The listing builds one solid part. Answer for the finished solid, in the listing's coordinates (mm). A direction names the side the tool comes from. Coordinates: 2 decimals unless noted, no trailing zeros. Order: outer loops, then holes, each group sorted by start corner. A loop starts at its lowest first (then second) coordinate and runs counter-clockwise, first axis right, second up. Notation, with made-up numbers: (24, -6) -> (34, -6) arc R10 ccw to (34, 10) -> close; hole circle Ø1 at (54.5, 16). An arc over 180 degrees is marked (long way). Write each question's results on one line, items separated by ' | '. Start each with the question number.
(1) Determine the mould class of faces 5 (the face through (10.75, -1.97, -25.84)), 6 (the face through (-10, 45, -205)), 7 (the face through (-5, -2, -169)), 8 (the face through (-33, -1, -126)) for opening direction X: +X half, -X half, draft (parallel to the pull), parting line (faces both ways), or undercut.
(2) A tool of negligible diameter and unlimited length cuts with its end or side. For faces 1 (the face through (-10, -2, -205)), 2 (the face through (3, 4, -207)), 3 (the face through (-5, -2, -13)), 4 (the face through (10.75, -1.97, -181.84)), from which of +Z, -Z, +X, -X, +Y, -Y can it reach the whole face along a straight path? Write none if from no direction.
(3) The part is cut by section D-D, the plane x = -17. Give the vertices of the cut face in (y, z).
(4) Given pin 1 (1.5 mm diameter, centred on x = -5.5, y = 38.5, fed in from +Z); pin 2 (6 mm diameter, centred on x = -15, z = -99, fed in from +Y), each flat-ended and moving along its own axis, determine where each tip first touches the part or whether it passes through.
(5) The part is cut by section C-C, the plane z = -66. Give the vertices of the cut face in (x, y).
(6) Straight lines are drawn through the part: L1, parallel to Y at x = 0, z = -200; L2, parallel to X at y = -3, z = 0; L3, parallel to Z at x = -6.5, y = 14. For each, find the intervals that lie inside material, in ascending order.
(7) The part is cut by section B-B, the plane y = 14. Give the vertices of the cut face in (x, z).
(8) The part is cut by section A-A, the plane x = 0. Give the vertices of the cut face in (y, z), then the cut area to 4 significant figures.
```python
from build123d import *

# Parameters (mm, degrees)
SKETCH5_W           = 26
SKETCH5_H           = 26
BOSS_EXTRUDE1_DEPTH = 10
SKETCH4_R           = 10.75
CUT_EXTRUDE1_DEPTH  = 4
SKETCH6_W           = 10
SKETCH6_H           = 3.483566845
CUT_EXTRUDE2_DEPTH  = 4
LPATTERN1_COUNT     = 8
LPATTERN1_PITCH     = 26
SKETCH7_W           = 10
SKETCH7_H           = 4
CUT_EXTRUDE3_DEPTH  = 183
SKETCH8_W           = 208
SKETCH8_H           = 10
BOSS_EXTRUDE2_DEPTH = 20
SKETCH9_W           = 46
SKETCH9_H           = 10
BOSS_EXTRUDE3_DEPTH = 20
SKETCH10_W          = 46
SKETCH10_H          = 20
BOSS_EXTRUDE4_DEPTH = 45
SKETCH13_W          = 20
SKETCH13_H          = 5
CUT_EXTRUDE4_DEPTH  = 20
SKETCH14_R          = 6
CUT_EXTRUDE5_DEPTH  = 45
SKETCH15_W          = 6
SKETCH15_H          = 19
CUT_EXTRUDE6_DEPTH  = 20


with BuildPart() as part:
    # Sketch5 → Boss-Extrude1 (new body)
    with BuildSketch(Plane(origin=(0, 0, 0), x_dir=(1, 0, 0), z_dir=(0, 1, 0))):
        Rectangle(SKETCH5_W, SKETCH5_H)
    boss_extrude1 = extrude(amount=-BOSS_EXTRUDE1_DEPTH)

    # Sketch4 → Cut-Extrude1 (cut)
    with BuildSketch(Plane(origin=(0, 0, 0), x_dir=(1, 0, 0), z_dir=(0, 1, 0))):
        Circle(SKETCH4_R)
    cut_extrude1 = extrude(amount=-CUT_EXTRUDE1_DEPTH, mode=Mode.SUBTRACT)

    # Sketch6 → Cut-Extrude2 (cut)
    with BuildSketch(Plane(origin=(0, 0, 0), x_dir=(1, 0, 0), z_dir=(0, 1, 0))):
        with Locations((0, 11.258216578)):
            Rectangle(SKETCH6_W, SKETCH6_H)
    cut_extrude2 = extrude(amount=-CUT_EXTRUDE2_DEPTH, mode=Mode.SUBTRACT)

    # LPattern1: Boss-Extrude1, Cut-Extrude1, Cut-Extrude2 ×8
    with Locations(*[(0, 0, -i * LPATTERN1_PITCH) for i in range(1, LPATTERN1_COUNT)]):
        add(boss_extrude1)
        add(cut_extrude1, mode=Mode.SUBTRACT)
        add(cut_extrude2, mode=Mode.SUBTRACT)

    # Sketch7 → Cut-Extrude3 (cut, through all)
    with BuildSketch(Plane.XY.offset(-13)):
        with Locations((0, -2)):
            Rectangle(SKETCH7_W, SKETCH7_H)
    extrude(amount=-CUT_EXTRUDE3_DEPTH, mode=Mode.SUBTRACT)

    # Sketch8 → Boss-Extrude2 (add)
    with BuildSketch(Plane.ZY.offset(13)):
        with Locations((-91, -5)):
            Rectangle(SKETCH8_W, SKETCH8_H)
    extrude(amount=BOSS_EXTRUDE2_DEPTH)

    # Sketch9 → Boss-Extrude3 (add)
    with BuildSketch(Plane(origin=(0, 0, -195), x_dir=(-1, 0, 0), z_dir=(0, 0, -1))):
        with Locations((10, -5)):
            Rectangle(SKETCH9_W, SKETCH9_H)
    extrude(amount=BOSS_EXTRUDE3_DEPTH)

    # Sketch10 → Boss-Extrude4 (add)
    with BuildSketch(Plane(origin=(0, 0, 0), x_dir=(1, 0, 0), z_dir=(0, 1, 0))):
        with Locations((-10, 205)):
            Rectangle(SKETCH10_W, SKETCH10_H)
    extrude(amount=BOSS_EXTRUDE4_DEPTH)

    # Sketch13 → Cut-Extrude4 (cut)
    with BuildSketch(Plane(origin=(0, 0, -215), x_dir=(-1, 0, 0), z_dir=(0, 0, -1))):
        with Locations((0, -1.5)):
            Rectangle(SKETCH13_W, SKETCH13_H)
    extrude(amount=-CUT_EXTRUDE4_DEPTH, mode=Mode.SUBTRACT)

    # Sketch14 → Cut-Extrude5 (cut)
    with BuildSketch(Plane(origin=(0, 0, -215), x_dir=(-1, 0, 0), z_dir=(0, 0, -1))):
        with Locations((0, 14)):
            Circle(SKETCH14_R)
    extrude(amount=-CUT_EXTRUDE5_DEPTH, mode=Mode.SUBTRACT)

    # Sketch15 → Cut-Extrude6 (cut)
    with BuildSketch(Plane(origin=(13, 0, 0), x_dir=(0, 0, -1), z_dir=(1, 0, 0))):
        with Locations((207, 13.5)):
            Rectangle(SKETCH15_W, SKETCH15_H)
    extrude(amount=-CUT_EXTRUDE6_DEPTH, mode=Mode.SUBTRACT)


solid = part.part
```
Established:
1) face 5: undercut | face 6: draft | face 7: undercut | face 8: -X half
2) face 1: -Z | face 2: +X | face 3: -Z, +Y | face 4: +Y
3) outline: (-10, -215) -> (45, -215) -> (45, -195) -> (0, -195) -> (0, 13) -> (-10, 13) -> close
4) pin 1: stops at z = -195 | pin 2: stops at y = 0
5) outline: (-33, -10) -> (13, -10) -> (13, 0) -> (5, 0) -> (5, -4) -> (-5, -4) -> (-5, 0) -> (-33, 0) -> close
6) L1: y = -10 to -4, 1 to 8, 20 to 45 | L2: x = -33 to -10.75, 10.75 to 13 | L3: z = -215 to -210, -204 to -195
7) outline: (-33, -215) -> (-6, -215) -> (-6, -210) -> (-7, -210) -> (-7, -204) -> (-6, -204) -> (-6, -195) -> (-33, -195) -> close; (6, -215) -> (13, -215) -> (13, -210) -> (6, -210) -> close; (6, -204) -> (13, -204) -> (13, -195) -> (6, -195) -> close
8) outline: (-10, -215) -> (-4, -215) -> (-4, 10.75) -> (0, 10.75) -> (0, 13) -> (-10, 13) -> close; (1, -215) -> (8, -215) -> (8, -210) -> (4, -210) -> (4, -204) -> (8, -204) -> (8, -195) -> (1, -195) -> close; (20, -215) -> (45, -215) -> (45, -195) -> (20, -195) -> (20, -204) -> (23, -204) -> (23, -210) -> (20, -210) -> close | area: 1,975 mm^2
